```python
from build123d import *

# Parameters (mm, degrees)
SKETCH1_R           = 1.7
BOSS_EXTRUDE1_DEPTH = 3
SKETCH2_W           = 11.3
SKETCH2_H           = 3
BOSS_EXTRUDE2_DEPTH = 29
SKETCH3_R           = 1.7
SKETCH3_R_2         = 2
CUT_EXTRUDE1_DEPTH  = 3
FILLET1_R           = 2
CHAMFER1_SIZE       = 1


with BuildPart() as part:
    # Sketch1 → Boss-Extrude1 (new body)
    with BuildSketch(Plane(origin=(0, 0, 0), x_dir=(1, 0, 0), z_dir=(0, 1, 0))):
        Polygon((5.65, 9.9), (-5.65, 9.9), (-5.65, -9.9), (5.65, -9.9), (5.65, -7.9), (8.65, -7.9), (8.65, 1.9), (5.65, 1.9), align=None)
        with Locations(Location((5, -3, 0), (0, 0, 270))):
            Circle(SKETCH1_R, mode=Mode.SUBTRACT)
    extrude(amount=BOSS_EXTRUDE1_DEPTH)

    # Sketch2 → Boss-Extrude2 (add)
    with BuildSketch(Plane(origin=(0, 3, 0), x_dir=(1, 0, 0), z_dir=(0, 1, 0))):
        with Locations((0, 8.4)):
            Rectangle(SKETCH2_W, SKETCH2_H)
    extrude(amount=BOSS_EXTRUDE2_DEPTH)

    # Sketch3 → Cut-Extrude1 (cut)
    with BuildSketch(Plane(origin=(0, 0, -9.9), x_dir=(-1, 0, 0), z_dir=(0, 0, -1))):
        with Locations((0, 28)):
            Circle(SKETCH3_R)
        with Locations((0, 10)):
            Circle(SKETCH3_R)
        with Locations((0, 19)):
            Circle(SKETCH3_R_2)
    extrude(amount=-CUT_EXTRUDE1_DEPTH, mode=Mode.SUBTRACT)

    # Fillet1
    fillet1_edges = [part.edges().sort_by_distance(p)[0] for p in [
        (0, 3, -6.9),
        (-5.65, 32, -8.4),
        (5.65, 32, -8.4),
    ]]
    fillet(fillet1_edges, radius=FILLET1_R)

    # Chamfer1
    chamfer1_edges = [part.edges().sort_by_distance(p)[0] for p in [
        (7.15, 3, -1.9),
        (0, 3, 9.9),
        (5.65, 3, 8.9),
        (7.15, 3, 7.9),
        (8.65, 3, 3),
        (5.65, 17.5, -6.9),
        (0, 32, -6.9),
        (-5.65, 17.5, -6.9),
        (-5.064213562, 31.414213562, -6.9),
        (5.064213562, 31.414213562, -6.9),
        (-5.65, 3, 2.5),
        (5.65, 3, -3.4),
        (5.65, 3.585786438, -6.314213562),
        (-5.65, 3.585786438, -6.314213562),
    ]]
    chamfer(chamfer1_edges, length=CHAMFER1_SIZE)


solid = part.part
```
The listing builds one solid part. Answer for the finished solid, in the listing's coordinates (mm). A direction names the side the tool comes from. Round coordinates to 2 decimals unless told otherwise and drop trailing zeros. Loops run counter-clockwise (first coordinate to the right, second up) from the corner with the lowest first, then second, coordinate; pieces in that order, holes last.
Q1. Given pin 1 Ø0.6 at (x, y) = (8, 0.5) entering from +Z; pin 2 Ø2.5 at (y, z) = (15, -7.5) entering from +X; pin 3 Ø6 at (x, y) = (1, 15) entering from +Z, each flat-ended and moving along its own axis, determine where each tip first touches the part or whether it passes through.
Q2. Section B-B, the plane y = 19 is taken. Determine the outline of the cut face in (x, z).
Q3. Section A-A, the plane z = 3 is taken. Determine the outline of the cut face in (x, y).
Q4. Which of the six approach directions +Z, -Z, +X, -X, +Y, -Y give full straight-line access (tool end or side, diameter ignored) to faces 4 (the face through (5.65, 12.7, -8.3)), 5 (the face through (-5.16, 17.67, -7.41)), 6 (the face through (6.7, 2.5, -1.4))?
Q5. Section D-D, the plane y = 7 is taken. Determine the outline of the cut face in (x, z).
Q6. Section C-C, the plane x = 0 is taken. Determine the outline of the cut face in (y, z), then the cut area to 3 significant figures.
Q7. For a pull along X with two mould halves and no side action, classify faces 1 (the face through (8.65, 1, 3)), 2 (the face through (0, 21, -8)), 3 (the face through (0, 16, -9.9)) as released by +X, released by -X, zero draft, split by the parting line, or undercut.
Q8. Find the intervals of material crossed by line 1 (Y direction, x = 0, z = -9); line 2 (Y direction, x = -0.25, z = 6.75); line 3 (Y direction, x = 0.5, z = -8.25), in increasing order.
Completed:
1. pin 1: stops at z = 7.9
1. pin 2: stops at x = 5.65
1. pin 3: stops at z = -6.9
2. outline: (-5.65, -9.9) - (-2, -9.9) - (-2, -6.9) - (-4.65, -6.9) - (-5.65, -7.9) - close; (2, -9.9) - (5.65, -9.9) - (5.65, -7.9) - (4.65, -6.9) - (2, -6.9) - close
3. outline: (-5.65, 0) - (3.3, 0) - (3.3, 3) - (-4.65, 3) - (-5.65, 2) - close; (6.7, 0) - (8.65, 0) - (8.65, 2) - (7.65, 3) - (6.7, 3) - close
4. face 4: -Z, +X, +Y, -Y
4. face 5: +Z, -X, +Y
4. face 6: +X, +Y
5. outline: (-5.65, -9.9) - (5.65, -9.9) - (5.65, -7.9) - (4.65, -6.9) - (-4.65, -6.9) - (-5.65, -7.9) - close
6. outline: (0, -9.9) - (8.3, -9.9) - (8.3, -6.9) - (5, -6.9) arc R2 cw to (3, -4.9) - (3, 8.9) - (2, 9.9) - (0, 9.9) - close; (11.7, -9.9) - (17, -9.9) - (17, -6.9) - (11.7, -6.9) - close; (21, -9.9) - (26.3, -9.9) - (26.3, -6.9) - (21, -6.9) - close; (29.7, -9.9) - (32, -9.9) - (32, -7.9) - (31, -6.9) - (29.7, -6.9) - close
6. area: 114 mm2
7. face 1: released by +X
7. face 2: undercut
7. face 3: zero draft
8. line 1: y = 0 to 8.3, 11.7 to 17, 21 to 26.3, 29.7 to 32
8. line 2: y = 0 to 3
8. line 3: y = 0 to 8.38, 11.62 to 17.06, 20.94 to 26.38, 29.62 to 32
